Could you check a few things on this model? Use its own coordinates, in mm. Round coordinates to 2 decimals unless told otherwise and drop trailing zeros. Loops run counter-clockwise (first coordinate to the right, second up) from the corner with the lowest first, then second, coordinate; pieces in that order, holes last. Notation, with made-up numbers: (74, 2.25) - (116, 2.25) arc R15 ccw to (116, 28.25) - close; hole circle Ø5 at (70.25, -35). An arc over 180 degrees is marked (long way). Use one line per item in the form item = value.
```python
from build123d import *
from OCP.BRepFilletAPI import BRepFilletAPI_MakeChamfer

# Parameters (mm, degrees)
BOSS_EXTRUDE1_DEPTH         = 2.54
SKETCH3_W                   = 0.635
SKETCH3_H                   = 0.635
CHAMFER1_SIZE               = 0.254
CHAMFER1_SIZE2              = 0.146646968
CHAMFER2_SIZE               = 0.127
CHAMFER2_SIZE2              = 0.219970453
LPATTERN1_COUNT             = 4
LPATTERN1_PITCH             = 2.54
CHAMFER1_OF_LPATTERN1_SIZE  = 0.254
CHAMFER1_OF_LPATTERN1_SIZE2 = 0.146646968
CHAMFER2_OF_LPATTERN1_SIZE2 = 0.127
CHAMFER2_OF_LPATTERN1_SIZE  = 0.219970453


with BuildPart() as part:
    # Sketch1 → Boss-Extrude1 (new body)
    with BuildSketch(Plane(origin=(0, 0, 0), x_dir=(1, 0, 0), z_dir=(0, 1, 0))):
        Polygon((1.016, 1.27), (1.27, 1.016), (1.27, -1.016), (1.016, -1.27), (-1.016, -1.27), (-1.27, -1.016), (-1.27, 1.016), (-1.016, 1.27), align=None)
    boss_extrude1 = extrude(amount=BOSS_EXTRUDE1_DEPTH)

    # Sweep1: sweep along a path in Sketch2
    with BuildLine(Plane.XY) as sweep1_path:
        Line((0, -2.921), (0, 0))
        Line((0, 0), (0, 8.2931))
    # Sketch3 → Sweep1 (sweep)
    with BuildSketch(Plane(origin=(0, -2.921, 0), x_dir=(-1, 0, 0), z_dir=(0, -1, 0))):
        Rectangle(SKETCH3_W, SKETCH3_H)
    sweep1 = sweep(path=sweep1_path.line)

    # Chamfer1: one chamfer whose edges measure the first distance from different faces: ONE call of the kernel's chamfer builder (chamfer() names one face for all edges)
    chamfer1_edges_1 = [part.edges().sort_by_distance(p)[0] for p in [
        (0.3175, -2.921, 0),
    ]]
    chamfer1_side_1 = [part.faces().sort_by_distance(p)[0] for p in [
        (0.3175, -1.4605, 0),
    ]]
    chamfer1_edges_2 = [part.edges().sort_by_distance(p)[0] for p in [
        (0, -2.921, 0.3175),
    ]]
    chamfer1_side_2 = [part.faces().sort_by_distance(p)[0] for p in [
        (0, -1.4605, 0.3175),
    ]]
    chamfer1_edges_3 = [part.edges().sort_by_distance(p)[0] for p in [
        (-0.3175, -2.921, 0),
    ]]
    chamfer1_side_3 = [part.faces().sort_by_distance(p)[0] for p in [
        (-0.3175, -1.4605, 0),
    ]]
    chamfer1_edges_4 = [part.edges().sort_by_distance(p)[0] for p in [
        (0, -2.921, -0.3175),
    ]]
    chamfer1_side_4 = [part.faces().sort_by_distance(p)[0] for p in [
        (0, -1.4605, -0.3175),
    ]]
    chamfer1 = BRepFilletAPI_MakeChamfer(part.part.solid().wrapped)
    for e in chamfer1_edges_1:
        chamfer1.Add(CHAMFER1_SIZE, CHAMFER1_SIZE2, e.wrapped, chamfer1_side_1[0].wrapped)  # the first distance lies on this face
    for e in chamfer1_edges_2:
        chamfer1.Add(CHAMFER1_SIZE, CHAMFER1_SIZE2, e.wrapped, chamfer1_side_2[0].wrapped)  # the first distance lies on this face
    for e in chamfer1_edges_3:
        chamfer1.Add(CHAMFER1_SIZE, CHAMFER1_SIZE2, e.wrapped, chamfer1_side_3[0].wrapped)  # the first distance lies on this face
    for e in chamfer1_edges_4:
        chamfer1.Add(CHAMFER1_SIZE, CHAMFER1_SIZE2, e.wrapped, chamfer1_side_4[0].wrapped)  # the first distance lies on this face
    add(Compound.cast(chamfer1.Shape()), mode=Mode.REPLACE)

    # Chamfer2
    chamfer2_edges = [part.edges().sort_by_distance(p)[0] for p in [
        (0.3175, 8.2931, 0),
        (0, 8.2931, 0.3175),
        (-0.3175, 8.2931, 0),
        (0, 8.2931, -0.3175),
    ]]
    chamfer2_side = [part.faces().sort_by_distance(p)[0] for p in [
        (0, 8.2931, 0),
    ]]
    chamfer(chamfer2_edges, length=CHAMFER2_SIZE, length2=CHAMFER2_SIZE2, reference=chamfer2_side[0])

    # LPattern1: Boss-Extrude1, Sweep1 ×4
    with Locations(*[(0, 0, i * LPATTERN1_PITCH) for i in range(1, LPATTERN1_COUNT)]):
        add(boss_extrude1)
        add(sweep1)

    # Chamfer1 of LPattern1: one chamfer whose edges measure the first distance from different faces: ONE call of the kernel's chamfer builder (chamfer() names one face for all edges)
    chamfer1_of_lpattern1_edges_1 = [part.edges().sort_by_distance(p)[0] for p in [
        (0.3175, -2.921, 2.54),
    ]]
    chamfer1_of_lpattern1_side_1 = [part.faces().sort_by_distance(p)[0] for p in [
        (0.3175, -1.4605, 2.54),
    ]]
    chamfer1_of_lpattern1_edges_2 = [part.edges().sort_by_distance(p)[0] for p in [
        (0, -2.921, 2.8575),
    ]]
    chamfer1_of_lpattern1_side_2 = [part.faces().sort_by_distance(p)[0] for p in [
        (0, -1.4605, 2.8575),
    ]]
    chamfer1_of_lpattern1_edges_3 = [part.edges().sort_by_distance(p)[0] for p in [
        (-0.3175, -2.921, 2.54),
    ]]
    chamfer1_of_lpattern1_side_3 = [part.faces().sort_by_distance(p)[0] for p in [
        (-0.3175, -1.4605, 2.54),
    ]]
    chamfer1_of_lpattern1_edges_4 = [part.edges().sort_by_distance(p)[0] for p in [
        (0, -2.921, 2.2225),
    ]]
    chamfer1_of_lpattern1_side_4 = [part.faces().sort_by_distance(p)[0] for p in [
        (0, -1.4605, 2.2225),
    ]]
    chamfer1_of_lpattern1_edges_5 = [part.edges().sort_by_distance(p)[0] for p in [
        (0.3175, -2.921, 5.08),
    ]]
    chamfer1_of_lpattern1_side_5 = [part.faces().sort_by_distance(p)[0] for p in [
        (0.3175, -1.4605, 5.08),
    ]]
    chamfer1_of_lpattern1_edges_6 = [part.edges().sort_by_distance(p)[0] for p in [
        (0, -2.921, 5.3975),
    ]]
    chamfer1_of_lpattern1_side_6 = [part.faces().sort_by_distance(p)[0] for p in [
        (0, -1.4605, 5.3975),
    ]]
    chamfer1_of_lpattern1_edges_7 = [part.edges().sort_by_distance(p)[0] for p in [
        (-0.3175, -2.921, 5.08),
    ]]
    chamfer1_of_lpattern1_side_7 = [part.faces().sort_by_distance(p)[0] for p in [
        (-0.3175, -1.4605, 5.08),
    ]]
    chamfer1_of_lpattern1_edges_8 = [part.edges().sort_by_distance(p)[0] for p in [
        (0, -2.921, 4.7625),
    ]]
    chamfer1_of_lpattern1_side_8 = [part.faces().sort_by_distance(p)[0] for p in [
        (0, -1.4605, 4.7625),
    ]]
    chamfer1_of_lpattern1_edges_9 = [part.edges().sort_by_distance(p)[0] for p in [
        (0.3175, -2.921, 7.62),
    ]]
    chamfer1_of_lpattern1_side_9 = [part.faces().sort_by_distance(p)[0] for p in [
        (0.3175, -1.4605, 7.62),
    ]]
    chamfer1_of_lpattern1_edges_10 = [part.edges().sort_by_distance(p)[0] for p in [
        (0, -2.921, 7.9375),
    ]]
    chamfer1_of_lpattern1_side_10 = [part.faces().sort_by_distance(p)[0] for p in [
        (0, -1.4605, 7.9375),
    ]]
    chamfer1_of_lpattern1_edges_11 = [part.edges().sort_by_distance(p)[0] for p in [
        (-0.3175, -2.921, 7.62),
    ]]
    chamfer1_of_lpattern1_side_11 = [part.faces().sort_by_distance(p)[0] for p in [
        (-0.3175, -1.4605, 7.62),
    ]]
    chamfer1_of_lpattern1_edges_12 = [part.edges().sort_by_distance(p)[0] for p in [
        (0, -2.921, 7.3025),
    ]]
    chamfer1_of_lpattern1_side_12 = [part.faces().sort_by_distance(p)[0] for p in [
        (0, -1.4605, 7.3025),
    ]]
    chamfer1_of_lpattern1 = BRepFilletAPI_MakeChamfer(part.part.solid().wrapped)
    for e in chamfer1_of_lpattern1_edges_1:
        chamfer1_of_lpattern1.Add(CHAMFER1_OF_LPATTERN1_SIZE, CHAMFER1_OF_LPATTERN1_SIZE2, e.wrapped, chamfer1_of_lpattern1_side_1[0].wrapped)  # the first distance lies on this face
    for e in chamfer1_of_lpattern1_edges_2:
        chamfer1_of_lpattern1.Add(CHAMFER1_OF_LPATTERN1_SIZE, CHAMFER1_OF_LPATTERN1_SIZE2, e.wrapped, chamfer1_of_lpattern1_side_2[0].wrapped)  # the first distance lies on this face
    for e in chamfer1_of_lpattern1_edges_3:
        chamfer1_of_lpattern1.Add(CHAMFER1_OF_LPATTERN1_SIZE, CHAMFER1_OF_LPATTERN1_SIZE2, e.wrapped, chamfer1_of_lpattern1_side_3[0].wrapped)  # the first distance lies on this face
    for e in chamfer1_of_lpattern1_edges_4:
        chamfer1_of_lpattern1.Add(CHAMFER1_OF_LPATTERN1_SIZE, CHAMFER1_OF_LPATTERN1_SIZE2, e.wrapped, chamfer1_of_lpattern1_side_4[0].wrapped)  # the first distance lies on this face
    for e in chamfer1_of_lpattern1_edges_5:
        chamfer1_of_lpattern1.Add(CHAMFER1_OF_LPATTERN1_SIZE, CHAMFER1_OF_LPATTERN1_SIZE2, e.wrapped, chamfer1_of_lpattern1_side_5[0].wrapped)  # the first distance lies on this face
    for e in chamfer1_of_lpattern1_edges_6:
        chamfer1_of_lpattern1.Add(CHAMFER1_OF_LPATTERN1_SIZE, CHAMFER1_OF_LPATTERN1_SIZE2, e.wrapped, chamfer1_of_lpattern1_side_6[0].wrapped)  # the first distance lies on this face
    for e in chamfer1_of_lpattern1_edges_7:
        chamfer1_of_lpattern1.Add(CHAMFER1_OF_LPATTERN1_SIZE, CHAMFER1_OF_LPATTERN1_SIZE2, e.wrapped, chamfer1_of_lpattern1_side_7[0].wrapped)  # the first distance lies on this face
    for e in chamfer1_of_lpattern1_edges_8:
        chamfer1_of_lpattern1.Add(CHAMFER1_OF_LPATTERN1_SIZE, CHAMFER1_OF_LPATTERN1_SIZE2, e.wrapped, chamfer1_of_lpattern1_side_8[0].wrapped)  # the first distance lies on this face
    for e in chamfer1_of_lpattern1_edges_9:
        chamfer1_of_lpattern1.Add(CHAMFER1_OF_LPATTERN1_SIZE, CHAMFER1_OF_LPATTERN1_SIZE2, e.wrapped, chamfer1_of_lpattern1_side_9[0].wrapped)  # the first distance lies on this face
    for e in chamfer1_of_lpattern1_edges_10:
        chamfer1_of_lpattern1.Add(CHAMFER1_OF_LPATTERN1_SIZE, CHAMFER1_OF_LPATTERN1_SIZE2, e.wrapped, chamfer1_of_lpattern1_side_10[0].wrapped)  # the first distance lies on this face
    for e in chamfer1_of_lpattern1_edges_11:
        chamfer1_of_lpattern1.Add(CHAMFER1_OF_LPATTERN1_SIZE, CHAMFER1_OF_LPATTERN1_SIZE2, e.wrapped, chamfer1_of_lpattern1_side_11[0].wrapped)  # the first distance lies on this face
    for e in chamfer1_of_lpattern1_edges_12:
        chamfer1_of_lpattern1.Add(CHAMFER1_OF_LPATTERN1_SIZE, CHAMFER1_OF_LPATTERN1_SIZE2, e.wrapped, chamfer1_of_lpattern1_side_12[0].wrapped)  # the first distance lies on this face
    add(Compound.cast(chamfer1_of_lpattern1.Shape()), mode=Mode.REPLACE)

    # Chamfer2 of LPattern1
    chamfer2_of_lpattern1_edges = [part.edges().sort_by_distance(p)[0] for p in [
        (0.3175, 8.2931, 2.54),
        (0, 8.2931, 2.8575),
        (-0.3175, 8.2931, 2.54),
        (0, 8.2931, 2.2225),
        (0.3175, 8.2931, 5.08),
        (0, 8.2931, 5.3975),
        (-0.3175, 8.2931, 5.08),
        (0, 8.2931, 4.7625),
        (0.3175, 8.2931, 7.62),
        (0, 8.2931, 7.9375),
        (-0.3175, 8.2931, 7.62),
        (0, 8.2931, 7.3025),
    ]]
    chamfer(chamfer2_of_lpattern1_edges, length=CHAMFER2_OF_LPATTERN1_SIZE, length2=CHAMFER2_OF_LPATTERN1_SIZE2)


solid = part.part
```
1. If we section it at B-B, the plane y = 0.25: Write out the boundary of the cut face in (x, z).
Solution:
outline = (-1.27, -1.02) - (-1.02, -1.27) - (1.02, -1.27) - (1.27, -1.02) - (1.27, 1.02) - (1.02, 1.27) - (1.27, 1.52) - (1.27, 3.56) - (1.02, 3.81) - (1.27, 4.06) - (1.27, 6.1) - (1.02, 6.35) - (1.27, 6.6) - (1.27, 8.64) - (1.02, 8.89) - (-1.02, 8.89) - (-1.27, 8.64) - (-1.27, 6.6) - (-1.02, 6.35) - (-1.27, 6.1) - (-1.27, 4.06) - (-1.02, 3.81) - (-1.27, 3.56) - (-1.27, 1.52) - (-1.02, 1.27) - (-1.27, 1.02) - close
2. For P1, Ø0.7, axis at y = -1, z = 7.5, coming from the +X side; P2, Ø1.3, axis at x = 0, z = 6, coming from the +Y side; P3, Ø0.5, axis at x = 0, y = -1.5, coming from the +Z side, each with a flat end and sliding along its axis, tell me the tip position at first contact or that it passes through.
Solution:
P1 = 0.32
P2 = 8.16
P3 = 7.94
3. If we section it at D-D, the plane z = 8.25: Write out the boundary of the cut face in (x, y).
Solution:
outline = (-1.27, 0) - (1.27, 0) - (1.27, 2.54) - (-1.27, 2.54) - close
4. If we section it at C-C, the plane x = 0.45: Write out the boundary of the cut face in (y, z).
Solution:
outline = (0, -1.27) - (2.54, -1.27) - (2.54, 8.89) - (0, 8.89) - close
5. Please list where these lines run through material, in increasing order: line 1 along Z through (x, y) = (0.1, 5.5); line 2 along Y through (x, z) = (-0.4, 1); line 3 along X through (y, z) = (5.25, 2.5).
Solution:
line_1 = -0.32 to 0.32, 2.22 to 2.86, 4.76 to 5.4, 7.3 to 7.94
line_2 = 0 to 2.54
line_3 = -0.32 to 0.32
6. We'd pull the mould along Z, two halves only. Please class faces 1 (the face through (0, 1, -1.27)), 2 (the face through (0, 0, 4)), 3 (the face through (-1.27, 1, 5)): +Z half, -Z half, draft (parallel to the pull), parting line (faces both ways), or undercut.
Solution:
face_1 = -Z half
face_2 = undercut
face_3 = draft
7. If we section it at A-A, the plane y = 3.5: Write out the boundary of the cut face in (x, z).
Solution:
outline = (-0.32, -0.32) - (0.32, -0.32) - (0.32, 0.32) - (-0.32, 0.32) - close; (-0.32, 2.22) - (0.32, 2.22) - (0.32, 2.86) - (-0.32, 2.86) - close; (-0.32, 4.76) - (0.32, 4.76) - (0.32, 5.4) - (-0.32, 5.4) - close; (-0.32, 7.3) - (0.32, 7.3) - (0.32, 7.94) - (-0.32, 7.94) - close
